Study the drawing (mm; zero at the part's minimum x, y, z) and answer. A direction names the side the tool comes from. Round coordinates to 2 decimals unless told otherwise and drop trailing zeros. Order: outer loops, then holes, each group sorted by start corner. A loop starts at its lowest first (then second) coordinate and runs counter-clockwise, first axis right, second up. Notation, with made-up numbers: M 84,23.25 L 93,23.25 A32 ccw 93,52.25 Z; hole C 19,85 d11. An arc over 180 degrees is marked long. Put each result on its own line as item: value. Start each with the question number.
1. Consider line 1 (X direction, y = 19.25, z = 23); line 2 (Z direction, x = 45, y = 18.5); line 3 (X direction, y = 22.25, z = 23). Determine where each line is inside the solid, lowest interval first.
2. Each of these flat-tipped pins is pushed along its axis until it touches: pin 1 Ø12 at (x, y) = (80, 10) entering from -Z; pin 2 Ø1.5 at (y, z) = (19.5, 32) entering from +X; pin 3 Ø10 at (x, z) = (75, 26.5) entering from -Y. Where does it stop, or does it pass through?
3. Which of the six approach directions +Z, -Z, +X, -X, +Y, -Y give full straight-line access (tool end or side, diameter ignored) to the marked faces 1, 2, 3, 4 and 5?
4. The part is cut by section D-D (x = 16). Give the vertices of the cut face in (y, z), then the cut area to 3 significant figures.
5. The part is cut by section A-A (x = 45). Give the vertices of the cut face in (y, z).
6. The part is cut by section B-B (y = 15.5). Give the vertices of the cut face in (x, z), then the cut area to 3 significant figures.
7. The mould has two halves that part along X. Classify the marked faces 6, 7 and 8: +X half, -X half, draft (parallel to the pull), parting line (faces both ways), or undercut.
8. The part is cut by section C-C (y = 10.5). Give the vertices of the cut face in (x, z) (3 decimals), then the cut area to 3 significant figures.
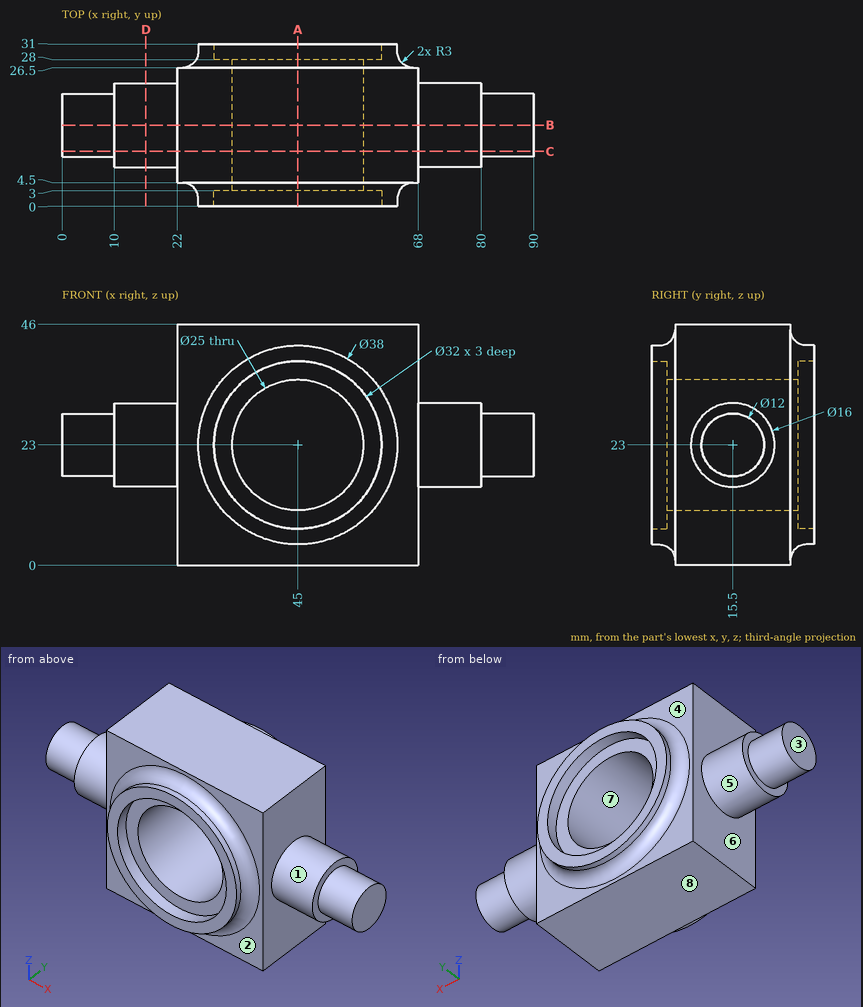
Resolved:
1. line 1: 0 to 32.5, 57.5 to 90
1. line 2: 0 to 10.5, 35.5 to 46
1. line 3: 10 to 32.5, 57.5 to 80
2. pin 1: z = 15
2. pin 2: x = 68
2. pin 3: y = 7.5
3. face 1: +X
3. face 2: -Y
3. face 3: +Z, -Z, -X, +Y, -Y
3. face 4: +Y
3. face 5: -X
4. outline: C 15.5,23 d16
4. area: 201 mm2
5. outline: M 0,4 L 1.5,4 A3 cw 4.5,1 L 4.5,0 L 26.5,0 L 26.5,1 A3 cw 29.5,4 L 31,4 L 31,7 L 28,7 L 28,10.5 L 3,10.5 L 3,7 L 0,7 Z; M 0,39 L 3,39 L 3,35.5 L 28,35.5 L 28,39 L 31,39 L 31,42 L 29.5,42 A3 cw 26.5,45 L 26.5,46 L 4.5,46 L 4.5,45 A3 cw 1.5,42 L 0,42 Z
6. outline: M 0,17 L 10,17 L 10,15 L 22,15 L 22,0 L 68,0 L 68,15 L 80,15 L 80,17 L 90,17 L 90,29 L 80,29 L 80,31 L 68,31 L 68,46 L 22,46 L 22,31 L 10,31 L 10,29 L 0,29 Z; hole C 45,23 d25
6. area: 2,250 mm2
7. face 6: -X half
7. face 7: undercut
7. face 8: draft
8. outline: M 0,19.683 L 10,19.683 L 10,16.755 L 22,16.755 L 22,0 L 68,0 L 68,16.755 L 80,16.755 L 80,19.683 L 90,19.683 L 90,26.317 L 80,26.317 L 80,29.245 L 68,29.245 L 68,46 L 22,46 L 22,29.245 L 10,29.245 L 10,26.317 L 0,26.317 Z; hole C 45,23 d25
8. area: 2,060 mm2
